Autodesk Inventor part; units mm, degrees
ref_plane "YZ Plane" through (0, 0, 0) normal (1, 0, 0) x (0, 1, 0)
ref_plane "XZ Plane" through (0, 0, 0) normal (0, 1, 0) x (-1, 0, 0)
ref_plane "XY Plane" through (0, 0, 0) normal (0, 0, 1) x (1, 0, 0)
sketch "スケッチ1" plane through (0, 0, 0) normal (0, 1, 0) x (-1, 0, 0)
  circle A0 centre (0, 0) radius 1.15
  circle A1 centre (0, 0) radius 2
  circle A2 centre (0, 0) radius 3.5
  line L0 (0, 0) -> (-3.5, 0)
  line L1 (-3.5, 0) -> (-3.5, 3.5)
  line L2 (-3.5, 3.5) -> (0, 3.5)
  line L3 (0, 3.5) -> (0, 0)
  line L4 (-2, 0) -> (2, 0)
  line L5 (2, 0) -> (2, -3.5)
  line L6 (2, -3.5) -> (-2, -3.5)
  line L7 (-2, -3.5) -> (-2, 0)
  line L8 (0, 0) -> (3.5, 0)
  line L9 (3.5, 0) -> (3.5, -4.5)
  line L10 (3.5, -4.5) -> (0, -4.5)
  line L11 (0, -4.5) -> (0, 0)
  line L12 (0, -3.5) -> (3.5, -4.5)
  line L13 (2, -3.5) -> (2, -4.5)
  point P0 (0, 2)
  point P1 (2, -2.8723)
  point P2 (2, -4.0714)
  dimension "d1" = 4
  dimension "d0" = 2.3
  dimension "d2" = 7
  dimension "d3" = 3.5
  dimension "d4" = 3.5
  dimension "d41" = 3.5
  dimension "d42" = 4.5
extrude "押し出し1" add sketch "スケッチ1" along normal blind 3.4 contours A1 L0 A2 L3
extrude "押し出し2" add sketch "スケッチ1" along normal blind 4.5 contours L8 A2 L5 | A1 L3 A2 L8 | A2 L9 L12 L13 L5
extrude "押し出し3" add sketch "スケッチ1" against normal blind 1 contours L4 A1 L11 A0 | A0 L3 A1 L4 | A0 L0 A1 L3 | L11 A1 L0 A0 | L5 A2 L11 A1 | L8 A2 L5 | A1 L3 A2 L8 | A1 L0 A2 L3 | L11 A2 L7 A1 | L7 A2 L0
sketch "スケッチ2" plane through (0, 4.5, 0) normal (0, 1, 0) x (1, 0, 0)
  circle A0 centre (0, 0) radius 1.15
  circle A1 centre (0, 0) radius 2
  circle A2 centre (0, 0) radius 3.5
  line L0 (2, 0) -> (-2, 0)
  line L1 (-2, 0) -> (-2, 3.5)
  line L2 (-2, 3.5) -> (2, 3.5)
  line L3 (2, 3.5) -> (2, 0)
  line L4 (-3.5, 4.5) -> (-3.5, 0)
  line L5 (0, 0) -> (-3.5, 0)
  line L6 (-3.5, 0) -> (-3.5, 4.5)
  line L7 (-3.5, 4.5) -> (0, 4.5)
  line L8 (0, 4.5) -> (0, 0)
  line L9 (0, 3.5) -> (-3.5, 4.5)
  line L10 (-2, 2.8723) -> (-2, 4.0714)
  line L11 (-2, 0) -> (-2, 4.0714)
  point P0 (0, 3.5)
  dimension "d12" = 4
  dimension "d11" = 2.3
  dimension "d13" = 7
  dimension "d14" = 4
  dimension "d15" = 3.5
  dimension "d43" = 3.5
  dimension "d44" = 4.5
extrude "押し出し4" add sketch "スケッチ2" along normal blind 1 contours L0 A1 A0 | A0 L8 A1 L0 | A0 L0 A1 L8 | L3 A2 L5 A1 | A1 L8 A2 L3 | A1 L1 A2 L8 | L5 A2 L1 | A2 L1 L2 | L2 L10 L9 | A2 L4 L9 L10 L1
sketch "スケッチ3" plane through (0, -1, 0) normal (0, -1, 0) x (1, 0, 0)
  circle A0 centre (0, 0) radius 1.15
  circle A1 centre (0, 0) radius 3.5
  line L0 (-3.5, 0) -> (3.5, 0)
  line L1 (3.5, 0) -> (3.5, 3.5)
  line L2 (3.5, 3.5) -> (-3.5, 3.5)
  line L3 (-3.5, 3.5) -> (-3.5, 0)
  line L4 (0, 0) -> (3.5, 0)
  line L5 (3.5, 0) -> (3.5, 3.5)
  line L6 (3.5, 3.5) -> (0, 3.5)
  line L7 (0, 3.5) -> (0, 0)
  line L8 (3.5, 0) -> (-3.5, 0)
  line L9 (-3.5, 0) -> (-3.5, 10)
  line L10 (-3.5, 10) -> (3.5, 10)
  line L11 (3.5, 10) -> (3.5, 0)
  line L12 (3.5, 10) -> (-1.5, 10)
  line L13 (-1.5, 10) -> (-1.5, 0)
  line L14 (-1.5, 0) -> (3.5, 0)
  line L15 (3.5, 0) -> (3.5, 10)
  line L16 (-3.5, 0) -> (-1.5, 0)
  line L17 (-1.5, 0) -> (-2.5, 0)
  line L18 (-2.5, 0) -> (-2.5, 10)
  circle A2 centre (0, 0) radius 3.25
  line L19 (0, 3.25) -> (3.5, 3.25)
  line L20 (3.5, 3.25) -> (3.5, 3.5)
  line L21 (3.5, 3.5) -> (0, 3.5)
  line L22 (0, 3.5) -> (0, 3.25)
  line L23 (0, 0) -> (-3.5, 0)
  line L24 (-3.5, 0) -> (-3.5, -4.5)
  line L25 (-3.5, -4.5) -> (0, -4.5)
  line L26 (0, -4.5) -> (0, 0)
  line L27 (0, -3.5) -> (-3.5, -4.5)
  point P0 (0, 3.5)
  point P1 (-1.5, 3.1623)
  point P2 (-2.5, 2.4495)
  point P3 (-2.5, 2.0767)
  dimension "d33" = 6.5
  dimension "d18" = 2.3
  dimension "d19" = 7
  dimension "d20" = 7
  dimension "d23" = 7
  dimension "d24" = 10
  dimension "d25" = 5
  dimension "d39" = 3.5
  dimension "d40" = 4.5
extrude "押し出し5" add sketch "スケッチ3" against normal blind 3.3 contours A1 L19 L1 | L2 L1 L19 A1 | L2 L13 L10 L11 | A1 L13 L2 | A1 L18 L2 L13 | L2 L18 L10 L13
extrude "押し出し6" add sketch "スケッチ3" along normal blind 2 contours A2 L13 A1 L7 | L7 A1 L19 | L2 L1 L19 A1 | L2 L13 L10 L11 | A1 L13 L2 | A2 L18 A1 L13 | A1 L18 L2 L13 | L2 L18 L10 L13
ref_plane "作業平面1" through (-2, 0, -3.5) normal (0, 0, 1) x (1, 0, 0)
sketch "スケッチ4" plane through (-2, 0, -3.5) normal (0, 0, 1) x (1, 0, 0)
  line L0 (2, 3.4) -> (2, 0)
  line L1 (2, 0) -> (2, 0.5)
  line L2 (2, 0.5) -> (0.5, 0.5)
  circle A0 centre (0.5, 0.5) radius 0.5
  line L3 (0, 0) -> (4, 0)
  dimension "d28" = 0.5
  dimension "d29" = 1.5
  dimension "d30" = 90
extrude "押し出し7" cut sketch "スケッチ4" along normal blind 20 contours A0
sketch "スケッチ5" plane through (-2.5, 2.3, 10) normal (0, 0, 1) x (1, 0, 0)
  line L0 (6, -3.3) -> (6, -5.3)
  line L1 (6, -5.3) -> (3.2, -5.3)
  line L2 (3.2, -5.3) -> (3.2, -2.8)
  line L3 (3.2, -2.8) -> (6, -2.8)
  line L4 (6, -2.8) -> (6, -5.3)
  circle A0 centre (3.2, -2.8) radius 1.4
  point P0 (2.5, -2.3)
  dimension "d34" = 2.8
  dimension "d35" = 2.5
  dimension "d36" = 2.8
extrude "押し出し8" cut sketch "スケッチ5" against normal blind 5 contours A0 L2 L3 | L3 L2 A0
extrude "押し出し9" add sketch "スケッチ3" against normal blind 1 contours L27 L24 A1
properties part number "trod2.0"
CAD build for the part. Positions are in the model's coordinates, mm. A direction names the side the tool comes from. Round coordinates to 2 decimals unless told otherwise and drop trailing zeros. Order: outer loops, then holes, each group sorted by start corner. A loop starts at its lowest first (then second) coordinate and runs counter-clockwise, first axis right, second up.
Item 1: Saw through at B-B on y = -0.5. Write the cut outline in (x, z).
Item 2: Pin check, flat tips, straight feed: pin 1 (3 mm diameter, centred on x = 1, y = 2.5, fed in from -Z); pin 2 (4.5 mm diameter, centred on y = 2.5, z = -3, fed in from +X); pin 3 (1.4 mm diameter, centred on x = 1, y = 0, fed in from +Z); pin 4 (1.8 mm diameter, centred on x = 0, z = 0, fed in from -Y). Stop position of each tip, or through.
Item 3: Saw through at C-C on z = 9.25. Write the cut outline in (x, y).
Item 4: Tool access for faces 1 (the face through (-1.44, 3.68, 3.19)), 2 (the face through (1, 0, -1)), 3 (the face through (-1.399, -1.986, 2.934)): list every direction of +Z, -Z, +X, -X, +Y, -Y with a clear straight run to the whole face (end or side of a thin tool).
Item 5: Mould opens along Z. For faces 4 (the face through (-0.91, 4.99, -0.7)), 5 (the face through (1, 0, 5)), 6 (the face through (-3.5, 2, -2)) say: pulls with the +Z half, pulls with the -Z half, needs draft (parallel to the pull), parting line crosses it, or undercut.
Item 6: Saw through at D-D on x = -1.75. Write the cut outline in (y, z), then the cut area to 3 significant figures.
Item 7: Saw through at A-A on x = 0.5. Write the cut outline in (y, z), then the cut area to 3 significant figures.
Item 8: Probe line 1 along Y through (x, z) = (0.7, 7.8); line 2 along Z through (x, y) = (0, -0.2); line 3 along Z through (x, y) = (0, 5.1). List the from-to ranges inside material, lowest first.
Reported:
1. outline: (-3.5, -4.5) - (0, -3.5) arc R3.5 ccw to (3.5, 0) - (3.5, 10) - (2.1, 10) - (2.1, 5) - (-0.7, 5) - (-0.7, 10) - (-2.5, 10) - (-2.5, 2.45) arc R3.5 ccw to (-3.5, 0) - close; hole circle Ø2.3 at (0, 0)
2. pin 1: stops at z = 0
2. pin 2: stops at x = 2.89
2. pin 3: stops at z = 5
2. pin 4: passes through
3. outline: (-2.5, -3) - (3.5, -3) - (3.5, 2.3) - (-2.5, 2.3) - close; hole circle Ø1 at (-1.5, 0.5); hole circle Ø2.8 at (0.7, -0.5)
4. face 1: +Y
4. face 2: -Z
4. face 3: -Z, +X, -Y
5. face 4: undercut
5. face 5: pulls with the +Z half
5. face 6: needs draft
6. outline: (-3, 2.74) - (-1, 2.74) - (-1, -4) - (0, -4) - (0, 0.97) - (0.07, 0.97) - (0.07, 10) - (-3, 10) - close; (0.93, 0.97) - (4.5, 0.97) - (4.5, -4) - (5.5, -4) - (5.5, 3.03) - (2.3, 3.03) - (2.3, 10) - (0.93, 10) - close
6. area: 53.0 mm2
7. outline: (-3, 3.25) - (-1, 3.25) - (-1, 1.04) - (0, 1.04) - (0, 1.94) - (3.4, 1.94) - (3.4, 3.46) - (2.3, 3.46) - (2.3, 10) - (0.89, 10) - (0.89, 5) - (-1.89, 5) - (-1.89, 10) - (-3, 10) - close; (-1, -3.46) - (0, -3.46) - (0, -1.04) - (-1, -1.04) - close; (4.5, -3.46) - (5.5, -3.46) - (5.5, -1.04) - (4.5, -1.04) - close; (4.5, 1.04) - (5.5, 1.04) - (5.5, 3.46) - (4.5, 3.46) - close
7. area: 36.1 mm2
8. line 1: y = -3 to -1.9, 0.9 to 2.3
8. line 2: z = -3.5 to -1.15, 1.15 to 5
8. line 3: z = -3.5 to -1.15, 1.15 to 3.5
